Autodesk Inventor part; units mm, degrees
ref_plane "YZ Plane" through (0, 0, 0) normal (1, 0, 0) x (0, 1, 0)
ref_plane "XZ Plane" through (0, 0, 0) normal (0, 1, 0) x (-1, 0, 0)
ref_plane "XY Plane" through (0, 0, 0) normal (0, 0, 1) x (1, 0, 0)
sketch "Sketch1" plane through (0, 0, 0) normal (0, 0, 1) x (1, 0, 0)
  line L0 (73.2079, 137.9474) -> (121.0158, 137.9474)
  line L1 (133.7158, 0) -> (73.2079, 0)
  line L2 (73.2079, 137.9474) -> (25.4, 137.9474)
  line L3 (25.4, 0) -> (73.2079, 0)
  line L4 (121.0158, 137.9474) -> (140.0658, 137.9474)
  arc A0 (146.4158, 131.5974) -> (140.0658, 137.9474) centre (140.0658, 131.5974) ccw
  line L5 (146.4158, 131.5974) -> (146.4158, 6.35)
  line L6 (25.4, 0) -> (6.35, 0)
  arc A1 (0, 6.35) -> (6.35, 0) centre (6.35, 6.35) ccw
  line L7 (0, 6.35) -> (0, 131.5974)
  arc A2 (6.35, 137.9474) -> (0, 131.5974) centre (6.35, 131.5974) ccw
  line L8 (6.35, 137.9474) -> (25.4, 137.9474)
  line L9 (140.0658, 0) -> (133.7158, 0)
  arc A3 (140.0658, 0) -> (146.4158, 6.35) centre (140.0658, 6.35) ccw
  arc A4 (9.525, 53.975) -> (9.525, 47.625) centre (9.525, 50.8) ccw
  arc A5 (15.875, 47.625) -> (15.875, 53.975) centre (15.875, 50.8) ccw
  line L10 (9.525, 53.975) -> (15.875, 53.975)
  line L11 (9.525, 47.625) -> (15.875, 47.625)
  arc A6 (9.525, 15.875) -> (9.525, 9.525) centre (9.525, 12.7) ccw
  arc A7 (15.875, 9.525) -> (15.875, 15.875) centre (15.875, 12.7) ccw
  line L12 (9.525, 15.875) -> (15.875, 15.875)
  line L13 (9.525, 9.525) -> (15.875, 9.525)
  arc A8 (130.5408, 53.975) -> (130.5408, 47.625) centre (130.5408, 50.8) ccw
  arc A9 (136.8908, 47.625) -> (136.8908, 53.975) centre (136.8908, 50.8) ccw
  line L14 (130.5408, 53.975) -> (136.8908, 53.975)
  line L15 (130.5408, 47.625) -> (136.8908, 47.625)
  arc A10 (130.5408, 15.875) -> (130.5408, 9.525) centre (130.5408, 12.7) ccw
  arc A11 (136.8908, 9.525) -> (136.8908, 15.875) centre (136.8908, 12.7) ccw
  line L16 (130.5408, 15.875) -> (136.8908, 15.875)
  line L17 (130.5408, 9.525) -> (136.8908, 9.525)
  arc A12 (84.5988, 62.6476) -> (90.9488, 62.6476) centre (87.7738, 62.6476) ccw
  arc A13 (90.9488, 68.9976) -> (84.5988, 68.9976) centre (87.7738, 68.9976) ccw
  line L18 (84.5988, 62.6476) -> (84.5988, 68.9976)
  line L19 (90.9488, 62.6476) -> (90.9488, 68.9976)
  circle A14 centre (133.7158, 125.2474) radius 2.54 construction
  circle A15 centre (133.7158, 87.1474) radius 2.54 construction
  arc A16 (79.7508, 61.6154) -> (59.4308, 61.6154) centre (69.5908, 61.6154) ccw
  arc A17 (59.4308, 55.2654) -> (79.7508, 55.2654) centre (69.5908, 55.2654) ccw
  line L20 (79.7508, 55.2654) -> (79.7508, 61.6154)
  line L21 (59.4308, 61.6154) -> (59.4308, 55.2654)
  point P0 (0, 0)
ref_plane "Work Plane1" through (0, 0, 6.35) normal (0, 0, 1) x (1, 0, 0)
sketch "Sketch3" plane through (0, 0, 6.35) normal (0, 0, 1) x (1, 0, 0)
  point P0 (0, 0)
  point P1 (133.7158, 87.1474)
  point P2 (133.7158, 125.2474)
extrude "Extrusion2" add sketch "Sketch1" along normal blind 6.35
hole "Hole1" at (133.7158, 87.1474, 6.35) at (133.7158, 125.2474, 6.35) direction (0, 0, -1) diameter 4.9784 depth 19.05 tip angle 118
properties part number "vrRig_v01r1_projMount"
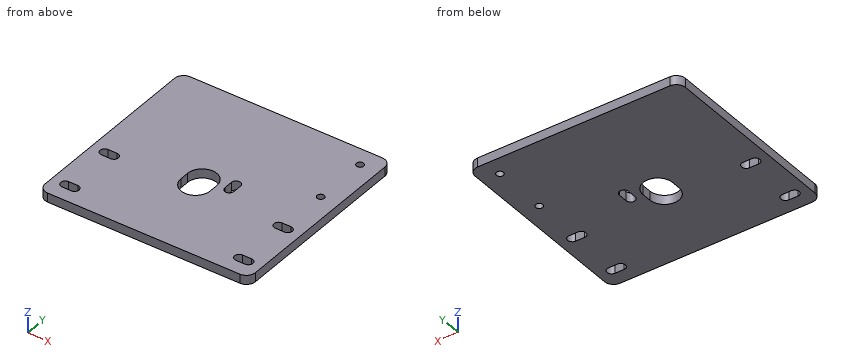
Here's how the part is built. I have some questions about the finished solid (model axes, mm). Give positions to 0.01 mm unless a question says otherwise; leave off trailing zeros. Order: outer loops, then holes, each group sorted by start corner. A loop starts at its lowest first (then second) coordinate and runs counter-clockwise, first axis right, second up. Notation, with made-up numbers: M 61.5,-5.5 L 65.5,-5.5 A28 ccw 65.5,30.5 Z; hole C 1.5,26 d9. An arc over 180 degrees is marked long. Use a Markdown table: item, result. Add a question column.
1. Suppose I cut it at C-C (z = 2.75). Give the number of separate pieces and of enclosed holes in the cut face, and give its area (3 significant figures).
2. I need wall thicknesses on probe 1 along Y at (x, z) = (14.5, 4) (3 decimals); probe 2 along X at (y, z) = (13, 2.5); probe 3 along Y at (x, z) = (18, 0.5). Which ranges of each line are inside material? Lowest first, please. Write a range as from..to.
3. Suppose I cut it at B-B (y = 50.8). List the corners of the cut face in (x, z) for me.
4. Suppose I cut it at D-D (y = 87). List the corners of the cut face in (x, z) for me.
5. Suppose I cut it at A-A (y = 12.7). List the corners of the cut face in (x, z) for me.
6. For pin 1 Ø3 at (x, y) = (133.72, 87.15) entering from +Z, with a flat end and sliding along its axis, tell me the tip position at first contact or that it passes through.
Results list:
| question | item | result |
|---|---|---|
| 1 | separate pieces | 1 |
| 1 | enclosed holes | 8 |
| 1 | area | 19,300 mm² |
| 2 | probe 1 | y = 0..9.525, 15.875..47.625, 53.975..137.947 |
| 2 | probe 2 | x = 0..6.36, 19.04..127.38, 140.05..146.42 |
| 2 | probe 3 | y = 0..10.34, 15.06..48.44, 53.16..137.95 |
| 3 | outline | M 0,0 L 6.35,0 L 6.35,6.35 L 0,6.35 Z; M 19.05,0 L 60.46,0 L 60.46,6.35 L 19.05,6.35 Z; M 78.72,0 L 127.37,0 L 127.37,6.35 L 78.72,6.35 Z; M 140.07,0 L 146.42,0 L 146.42,6.35 L 140.07,6.35 Z |
| 4 | outline | M 0,0 L 131.23,0 L 131.23,6.35 L 0,6.35 Z; M 136.2,0 L 146.42,0 L 146.42,6.35 L 136.2,6.35 Z |
| 5 | outline | M 0,0 L 6.35,0 L 6.35,6.35 L 0,6.35 Z; M 19.05,0 L 127.37,0 L 127.37,6.35 L 19.05,6.35 Z; M 140.07,0 L 146.42,0 L 146.42,6.35 L 140.07,6.35 Z |
| 6 | pin 1 | passes through |
